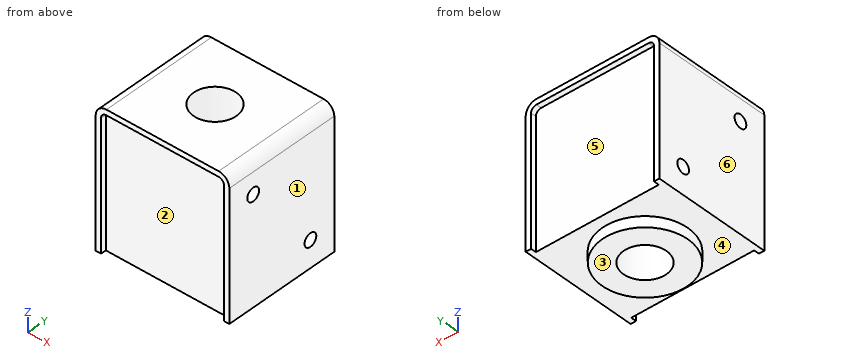
Autodesk Inventor part; units mm, degrees
ref_plane "YZ Plane" through (0, 0, 0) normal (1, 0, 0) x (0, 1, 0)
ref_plane "XY Plane" through (0, 0, 0) normal (0, 0, 1) x (1, 0, 0)
sketch "Sketch2" plane through (0, 0, 0) normal (0, 1, 0) x (-1, 0, 0)
  line L0 (-12.5, -13) -> (12.5, -13)
  line L1 (12.5, -13) -> (12.5, 13)
  line L2 (12.5, 13) -> (-12.5, 13)
  line L3 (-12.5, 13) -> (-12.5, -13)
  line L4 (-12.5, -13) -> (12.5, 13) construction
  line L5 (12.5, -13) -> (-12.5, 13) construction
  point P0 (0, 0)
  dimension "d0" = 25
  dimension "d1" = 26
extrude "Extrusion1" add sketch "Sketch2" along normal blind 22
sketch "Sketch3" plane through (12.5, 0, 13) normal (1, 0, 0) x (0, 0, -1)
  line L0 (0, 0) -> (26, 0)
  line L1 (0, 22) -> (26, 22)
  line L2 (0, 0) -> (0, 22)
  point P0 (13, 0)
  point P1 (6, 5)
  point P2 (21, 17)
  dimension "d4" = 12
  dimension "d5" = 5
  dimension "d6" = 5
  dimension "d7" = 6
  dimension "d8" = 15
hole "Hole1" at (12.5, 5, 7) at (12.5, 17, -8) direction (-1, 0, 0) diameter 2.459 depth 8.8
mirror "Mirror1" about plane through (0, 0, 0) normal (1, 0, 0) of "Hole1"
fillet "Fillet1" radius 2 2 edges at (12.5, 11, 13) (-12.5, 11, 13)
sketch "Sketch4" plane through (0, 22, 0) normal (0, 1, 0) x (1, 0, 0)
  arc A0 (-12.5, -11) -> (-10.5, -13) centre (-10.5, -11) ccw construction
  line L0 (-10.5, -13) -> (10.5, -13) construction
  arc A1 (10.5, -13) -> (12.5, -11) centre (10.5, -11) ccw construction
  line L1 (12.5, -11) -> (12.5, 13) construction
  line L2 (12.5, 13) -> (-12.5, 13) construction
  line L3 (-12.5, 13) -> (-12.5, -11) construction
  arc A2 (-11.5, -11) -> (-10.5, -12) centre (-10.5, -11) ccw
  line L4 (-10.5, -12) -> (10.5, -12)
  arc A3 (10.5, -12) -> (11.5, -11) centre (10.5, -11) ccw
  line L5 (11.5, -11) -> (11.5, 12)
  line L6 (11.5, 12) -> (-11.5, 12)
  line L7 (-11.5, 12) -> (-11.5, -11)
  line L8 (12.5, 13) -> (-12.5, 13)
  line L9 (-11.5, 12) -> (11.5, 12)
  line L10 (11.5, 12) -> (11.5, 13)
  line L11 (11.5, 13) -> (-11.5, 13)
  line L12 (-11.5, 13) -> (-11.5, 12)
  point P0 (0, 0)
  dimension "d17" = 1
extrude "Extrusion2" cut sketch "Sketch4" against normal blind 1
ref_plane "Work Plane1" through (0, 11, 0) normal (0, 1, 0) x (-1, 0, 0)
mirror "Mirror2" about plane through (0, 11, 0) normal (0, 1, 0) of "Extrusion2"
sketch "Sketch5" plane through (-12.5, 0, -13) normal (0, 0, -1) x (-1, 0, 0)
  line L0 (-25, 0) -> (-25, 22) construction
  line L1 (0, 0) -> (0, 22) construction
  line L2 (-25, 0) -> (0, 22) construction
  line L3 (-25, 22) -> (-24, 22) construction
  line L4 (-25, 22) -> (0, 0) construction
  circle A0 centre (-12.5, 11) radius 8
  point P0 (-12.5, 0)
  dimension "d21" = 16
extrude "Extrusion3" add sketch "Sketch5" along normal blind 2
sketch "Sketch6" plane through (0, 11, -15) normal (0, 0, -1) x (-1, 0, 0)
  circle A0 centre (0, 0) radius 4
  point P0 (0, -11)
  dimension "d24" = 8
extrude "Extrusion4" cut sketch "Sketch6" against normal through all
properties part number "main_block"
CAD build for the part. Positions are in the model's coordinates, mm. Face numbers are marked on the shaded views. A direction names the side the tool comes from. Round coordinates to 2 decimals unless told otherwise and drop trailing zeros. Write each loop counter-clockwise with the first axis right and the second up, starting at its lowest first coordinate (ties: lowest second). Pieces come first, ordered by that corner, then holes. Notation, with made-up numbers: M -15,83 L 31,83 A29 cw 31,110 Z; hole C 52.5,61 d8. An arc over 180 degrees is marked long. One line per question, with ' | ' between items.
1. Pin check, flat tips, straight feed: pin 1 Ø3 at (x, z) = (-9.5, 6) entering from +Y; pin 2 Ø0.5 at (x, y) = (-2.5, 0.5) entering from -Z; pin 3 Ø2 at (x, z) = (5, 6.5) entering from -Y. Stop position of each tip, or through.
Working result:
pin 1: y = 21 | pin 2: z = 12 | pin 3: y = 1
2. Cut at B-B on x = 0. Write the cut outline in (y, z), and give its area (3 significant figures).
Working result:
outline: M 0,12 L 1,12 L 1,-13 L 3,-13 L 3,-15 L 7,-15 L 7,13 L 0,13 Z; M 15,-15 L 19,-15 L 19,-13 L 21,-13 L 21,12 L 22,12 L 22,13 L 15,13 Z | area: 330 mm2
3. Cut at C-C on y = 11. Write the cut outline in (x, z).
Working result:
outline: M -12.5,-13 L -8,-13 L -8,-15 L -4,-15 L -4,13 L -10.5,13 A2 ccw -12.5,11 Z; M 4,-15 L 8,-15 L 8,-13 L 12.5,-13 L 12.5,11 A2 ccw 10.5,13 L 4,13 Z
4. Cut at A-A on z = -8. Write the cut outline in (x, y), and give its area (3 significant figures).
Working result:
outline: M -12.5,0 L -11.5,0 L -11.5,1 L 11.5,1 L 11.5,0 L 12.5,0 L 12.5,15.77 L 3.7,15.77 L 3.7,18.23 L 12.5,18.23 L 12.5,22 L 11.5,22 L 11.5,21 L -11.5,21 L -11.5,22 L -12.5,22 L -12.5,18.23 L -3.7,18.23 L -3.7,15.77 L -12.5,15.77 Z; hole C 0,11 d8 | area: 410 mm2
5. Probe L1, parallel to Y at x = 9, z = 7; L2, parallel to Y at x = -9.5, z = -8; L3, parallel to Z at x = -7.75, y = 17. List the from-to ranges inside material, lowest first. Write a range as from..to.
Working result:
L1: 1..3.77, 6.23..21 | L2: 1..15.77, 18.23..21 | L3: -13..-9.23, -6.77..13
6. Cut at D-D on x = -9.25. Write the cut outline in (y, z).
Working result:
outline: M 0,12 L 1,12 L 1,-13 L 21,-13 L 21,12 L 22,12 L 22,13 L 0,13 Z; hole C 5,7 d2.46; hole C 17,-8 d2.46
7. Which spindle directions (+Z, -Z, +X, -X, +Y, -Y) get a long thin tool onto all of the face, cutting with end or side? Do the marked faces 4, 5 and 6. Say none if no direction does.
Working result:
face 4: -Z | face 5: -Z, +Y | face 6: +Z, -Z, -X, +Y, -Y
8. Mould opens along X. For the marked faces 1, 2 and 3 say: pulls with the +X half, pulls with the -X half, needs draft (parallel to the pull), parting line crosses it, or undercut.
Working result:
face 1: pulls with the +X half | face 2: undercut | face 3: needs draft
